from build123d import *

# Parameters (mm, degrees)
SKETCH_W             = 25.4
SKETCH_H             = 3.175
PAD_DEPTH            = 25.4
SKETCH001_W          = 28.575
SKETCH001_H          = 12.7
PAD001_DEPTH         = 1.81
PAD001_DEPTH_BACK    = 5.715
POCKET_DEPTH         = 9.525
POCKET001_DEPTH      = 12.7
CHAMFER_SIZE         = 1.8034
SKETCH004_R          = 3.2512
POCKET002_DEPTH      = 5.716
PAD002_DEPTH         = 10.795
FILLET_R             = 4.953
SKETCH013_W          = 11.37
SKETCH013_H          = 12.7
SKETCH013_R          = 1.6002
PAD008_DEPTH         = 20.955
POCKET003_DEPTH      = 8.1961
SKETCH014_W          = 2.9
SKETCH014_H          = 10.2288
POCKET004_DEPTH      = 7.65
SKETCH015_W          = 2.9
SKETCH015_H          = 5.8
POCKET005_DEPTH      = 9.8644
SKETCH016_R          = 0.65
SKETCH016_W          = 0.825
SKETCH016_H          = 1.173477
POCKET006_DEPTH      = 6.5866
SKETCH017_R          = 0.65
SKETCH017_W          = 0.825
SKETCH017_H          = 1.173477
POCKET007_DEPTH      = 7.5866
POCKET007_DEPTH_BACK = 20.9904
SKETCH018_R          = 1.6002
SKETCH019_R          = 3.175
SKETCH020_W          = 25.4
SKETCH020_H          = 6.35
POCKET008_DEPTH      = 2.54
FILLET001_R          = 2.286


with BuildPart() as part:
    # Sketch → Pad (new body)
    with BuildSketch(Plane.XY):
        with Locations((-12.7, 1.5875)):
            Rectangle(SKETCH_W, SKETCH_H)
    extrude(amount=PAD_DEPTH)

    # Sketch001 (on Face1 of Pad) → Pad001 (join, two sides)
    with BuildSketch(Plane(origin=(0, 3.175, 0), x_dir=(-1, 0, 0), z_dir=(0, 1, 0))) as pad001_sk:
        with Locations((-14.2875, 12.7)):
            Rectangle(SKETCH001_W, SKETCH001_H)
    extrude(amount=PAD001_DEPTH)
    extrude(pad001_sk.sketch, amount=-PAD001_DEPTH_BACK)

    # Sketch002 (on Face13 of Pad001) → Pocket (cut)
    with BuildSketch(Plane.YZ.offset(28.575)):
        Polygon((9.150137, 19.05), (2.800137, 12.7), (9.150137, 6.35), align=None)
    extrude(amount=-POCKET_DEPTH, mode=Mode.SUBTRACT)

    # Sketch003 (on Face16 of Pocket) → Pocket001 (cut)
    with BuildSketch(Plane.YZ.offset(19.05)):
        with BuildLine():
            ThreePointArc((4.08, 14.732), (2.048, 12.7), (4.08, 10.668))
            Line((4.985, 10.668), (4.08, 10.668))
            Line((4.985, 14.732), (4.985, 10.668))
            Line((4.08, 14.732), (4.985, 14.732))
        make_face()
    extrude(amount=-POCKET001_DEPTH, mode=Mode.SUBTRACT)

    # Chamfer
    chamfer_edges = [part.edges().sort_by_distance(p)[0] for p in [
        (0, 4.985, 12.7),
    ]]
    chamfer(chamfer_edges, length=CHAMFER_SIZE)

    # Sketch004 (on Face4 of Chamfer) → Pocket002 (cut, through all)
    with BuildSketch(Plane(origin=(0, 3.175, 0), x_dir=(-1, 0, 0), z_dir=(0, 1, 0))):
        with Locations((12.7, 12.7)):
            Circle(SKETCH004_R)
    extrude(amount=-POCKET002_DEPTH, mode=Mode.SUBTRACT)

    # Sketch006 (on Face4 of Pocket002) → Pad002 (join)
    with BuildSketch(Plane(origin=(0, 3.175, 0), x_dir=(-1, 0, 0), z_dir=(0, 1, 0))):
        Polygon((0, 0), (-3.175, 0), (-3.175, 28.575), (25.4, 28.575), (25.4, 25.4), (0, 25.4), align=None)
    extrude(amount=-PAD002_DEPTH)

    # Fillet
    fillet_edges = [part.edges().sort_by_distance(p)[0] for p in [
        (3.175, -2.54, 12.7),
    ]]
    fillet(fillet_edges, radius=FILLET_R)

    # Sketch013 (on Face4 of Fillet) → Pad008 (join)
    with BuildSketch(Plane.YZ.offset(28.575)):
        with Locations((3.145, 12.7)):
            Rectangle(SKETCH013_W, SKETCH013_H)
        with Locations((4.08, 12.7)):
            Circle(SKETCH013_R, mode=Mode.SUBTRACT)
    extrude(amount=PAD008_DEPTH)

    # Pad008 Face13 → Pocket003 (cut)
    with BuildSketch(Plane(origin=(28.575, 6.929443, 12.7), x_dir=(0, 1, 0), z_dir=(-1, 0, 0))):
        with BuildLine():
            Line((-1.944443, -2.184863), (-1.944443, -6.35))
            Line((-1.944443, -6.35), (1.900557, -6.35))
            Line((1.900557, -6.35), (1.900557, 6.35))
            Line((1.900557, 6.35), (-1.944443, 6.35))
            Line((-1.944443, 6.35), (-1.944443, 2.184863))
            Line((-1.944443, 2.184863), (-2.556204, 1.573102))
            ThreePointArc((-2.556204, 1.573102), (-1.618614, 1.022594), (-1.249243, 0))
            ThreePointArc((-1.249243, 0), (-1.618614, -1.022594), (-2.556204, -1.573102))
            Line((-2.556204, -1.573102), (-1.944443, -2.184863))
        make_face()
    extrude(amount=-POCKET003_DEPTH, mode=Mode.SUBTRACT)

    # Sketch014 (on Face15 of Pocket003) → Pocket004 (cut)
    with BuildSketch(Plane(origin=(0, 8.83, 0), x_dir=(-1, 0, 0), z_dir=(0, 1, 0))):
        with Locations((-46.325, 12.7)):
            Rectangle(SKETCH014_W, SKETCH014_H)
    extrude(amount=-POCKET004_DEPTH, mode=Mode.SUBTRACT)

    # Sketch015 (on Face15 of Pocket004) → Pocket005 (cut)
    with BuildSketch(Plane(origin=(0, 8.83, 0), x_dir=(-1, 0, 0), z_dir=(0, 1, 0))):
        with Locations((-40.5108, 12.7)):
            Rectangle(SKETCH015_W, SKETCH015_H)
    extrude(amount=-POCKET005_DEPTH, mode=Mode.SUBTRACT)

    # Sketch016 (on Face53 of Pocket005) → Pocket006 (cut, through all)
    with BuildSketch(Plane(origin=(0, -1.0344, 0), x_dir=(-1, 0, 0), z_dir=(0, 1, 0))):
        with Locations((-39.79856, 12.7)):
            Circle(SKETCH016_R)
        with Locations((-41.58606, 15.013261)):
            Rectangle(SKETCH016_W, SKETCH016_H)
        with Locations((-41.58606, 10.386738)):
            Rectangle(SKETCH016_W, SKETCH016_H)
        with Locations((-39.51106, 15.013261)):
            Rectangle(SKETCH016_W, SKETCH016_H)
        with Locations((-39.51106, 10.386738)):
            Rectangle(SKETCH016_W, SKETCH016_H)
    extrude(amount=-POCKET006_DEPTH, mode=Mode.SUBTRACT)

    # Sketch017 (on Face52 of Pocket006) → Pocket007 (cut, two sides)
    with BuildSketch(Plane.XY.offset(7.5856)) as pocket007_sk:
        with Locations((45.57522, 4.07924)):
            Circle(SKETCH017_R)
        with Locations((45.2875, 6.392501)):
            Rectangle(SKETCH017_W, SKETCH017_H)
        with Locations((45.2875, 1.765978)):
            Rectangle(SKETCH017_W, SKETCH017_H)
        with Locations((47.3625, 6.392501)):
            Rectangle(SKETCH017_W, SKETCH017_H)
        with Locations((47.3625, 1.765978)):
            Rectangle(SKETCH017_W, SKETCH017_H)
    extrude(amount=-POCKET007_DEPTH, mode=Mode.SUBTRACT)
    extrude(pocket007_sk.sketch, amount=POCKET007_DEPTH_BACK, mode=Mode.SUBTRACT)

    # Sketch018 (on Face12 of Pocket007) → SubtractiveLoft section 0
    with BuildSketch(Plane(origin=(36.7711, 0, 0), x_dir=(0, -1, 0), z_dir=(-1, 0, 0))):
        with Locations((-4.07924, 12.7)):
            Circle(SKETCH018_R)
    # Sketch019 (on Face87 of Pocket007) → SubtractiveLoft section 1
    with BuildSketch(Plane.YZ.offset(28.575)):
        with Locations((4.07924, 12.7)):
            Circle(SKETCH019_R)
    loft(mode=Mode.SUBTRACT)

    # Sketch020 (on Face2 of SubtractiveLoft) → Pocket008 (cut)
    with BuildSketch(Plane.XZ.offset(2.54)):
        with Locations((24.003, 12.7)):
            Rectangle(SKETCH020_W, SKETCH020_H)
    extrude(amount=-POCKET008_DEPTH, mode=Mode.SUBTRACT)

    # Fillet001
    fillet001_edges = [part.edges().sort_by_distance(p)[0] for p in [
        (24.003, 0, 15.875),
        (36.703, 0, 12.7),
        (24.003, 0, 9.525),
        (11.303, 0, 12.7),
    ]]
    fillet(fillet001_edges, radius=FILLET001_R)


solid = part.part
CAD build for the part. Positions are in the model's coordinates, mm. A direction names the side the tool comes from. Coordinates: 2 decimals unless noted, no trailing zeros. Write each loop counter-clockwise with the first axis right and the second up, starting at its lowest first coordinate (ties: lowest second). Pieces come first, ordered by that corner, then holes. Notation, with made-up numbers: M 71,-29.75 L 117,-29.75 A24 cw 117,-18.75 Z; hole C -6.5,41.5 d2. An arc over 180 degrees is marked long. Answer as a JSON object with one key per item and string values. Group by question number.
1) Saw through at D-D (z = 19.75). Write the cut outline in (x, y) (3 decimals).
2) Tool access for faces 1 (the face through (29, -2.54, 17)), 2 (the face through (46, 5, 7.586)), 3 (the face through (37.9, 3.73, 11.14)): list every direction of +Z, -Z, +X, -X, +Y, -Y with a clear straight run to the whole face (end or side of a thin tool).
3) Saw through at B-B (x = 43.5). Write the cut outline in (y, z).
4) Mould opens along X. For faces 4 (the face through (-8.1, 0.3, 0)), 5 (the face through (41, -1.034, 13)), 6 (the face through (-25.4, 1, 17)) say: +X half, -X half, draft (parallel to the pull), parting line (faces both ways), or undercut.
5) Pin check, flat tips, straight feed: pin 1 Ø1 at (y, z) = (-1.5, 19) entering from -X; pin 2 Ø6 at (x, y) = (7, -1) entering from +Z; pin 3 Ø7.5 at (x, z) = (-12, 18) entering from -Y; pin 4 Ø3 at (x, y) = (-5, -1) entering from -Z. Stop position of each tip, or through.
6) Saw through at C-C (y = -6). Write the cut outline in (x, z) (3 decimals), plus the area to 3 significant figures.
7) Saw through at A-A (x = -12.7). Write the cut outline in (y, z) (3 decimals), plus the area to 3 significant figures.
8) Wall check: line 1 (X direction, y = 6.5, z = 9.5) (3 decimals); line 2 (Y direction, x = 48.5, z = 12.7); line 3 (X direction, y = 6.75, z = 11.5) (3 decimals). Give the ranges that are in metal, low to high. Write a range as from..to.
Values follow:
{
 "1": {"outline": "M -25.4,0 L 0,0 L 0,-7.62 L 3.175,-7.62 L 3.175,3.175 L -25.4,3.175 Z"},
 "2": {"face 1": "+Z, -Z, +X, -Y", "face 2": "+Y", "face 3": "+X"},
 "3": {"outline": "M -2.54,6.35 L 8.83,6.35 L 8.83,19.05 L -2.54,19.05 Z; hole C 4.08,12.7 d3.2"},
 "4": {"face 4": "draft", "face 5": "undercut", "face 6": "-X half"},
 "5": {"pin 1": "stops at x = 0", "pin 2": "stops at z = 19.05", "pin 3": "stops at y = 0", "pin 4": "stops at z = 0"},
 "6": {"outline": "M -25.4,25.4 L 0,25.4 L 0,0 L 3.175,0 L 3.175,6.35 L 3.405,6.35 L 3.405,19.05 L 3.175,19.05 L 3.175,28.575 L -25.4,28.575 Z", "area": "174 mm2"},
 "7": {"outline": "M -7.62,25.4 L 0,25.4 L 0,15.951 L 3.175,15.951 L 3.175,28.575 L -7.62,28.575 Z; M 0,0 L 3.175,0 L 3.175,9.449 L 0,9.449 Z", "area": "94.3 mm2"},
 "8": {"line 1": "x = 36.771..44.875, 47.775..49.53", "line 2": "y = -2.54..2.48, 5.68..8.83", "line 3": "x = 36.771..39.061, 41.961..44.875, 47.775..49.53"}
}
